Here's how the part is built. I have some questions about the finished solid (model axes, mm). Face numbers are marked on the shaded views. A direction names the side the tool comes from. Round coordinates to 2 decimals unless told otherwise and drop trailing zeros. Order: outer loops, then holes, each group sorted by start corner. A loop starts at its lowest first (then second) coordinate and runs counter-clockwise, first axis right, second up. Notation, with made-up numbers: M 33.25,-40 L 83.25,-40 A28 ccw 83.25,-7 Z; hole C -36.5,15.5 d2. An arc over 180 degrees is marked long. Write each question's results on one line, items separated by ' | '. Start each with the question number.
```python
from build123d import *

# Parameters (mm, degrees)
SKETCH1_R           = 9
SKETCH1_R_2         = 4
BOSS_EXTRUDE1_DEPTH = 5
SKETCH2_W           = 5
SKETCH2_H           = 10
CUT_EXTRUDE3_DEPTH  = 4
CIRPATTERN1_COUNT   = 6


with BuildPart() as part:
    # Sketch1 → Boss-Extrude1 (new body, symmetric)
    with BuildSketch(Plane.XY):
        Circle(SKETCH1_R)
        Circle(SKETCH1_R_2, mode=Mode.SUBTRACT)
    extrude(amount=BOSS_EXTRUDE1_DEPTH, both=True)

    # Sketch2 → Cut-Extrude3 (cut)
    with BuildSketch(Plane(origin=(-9, -17.193061184, 0), x_dir=(0, -1, 0), z_dir=(1, 0, 0))):
        with Locations((-17.193061184, 0)):
            Rectangle(SKETCH2_W, SKETCH2_H)
    cut_extrude3 = extrude(amount=CUT_EXTRUDE3_DEPTH, mode=Mode.SUBTRACT)

    # CirPattern1: Cut-Extrude3 ×6 about axis
    cirpattern1_axis = Axis((0, 0, 0), (0, 0, 1))
    for i in range(1, CIRPATTERN1_COUNT):
        add(cut_extrude3.rotate(cirpattern1_axis, i * 360 / CIRPATTERN1_COUNT), mode=Mode.SUBTRACT)


solid = part.part
```
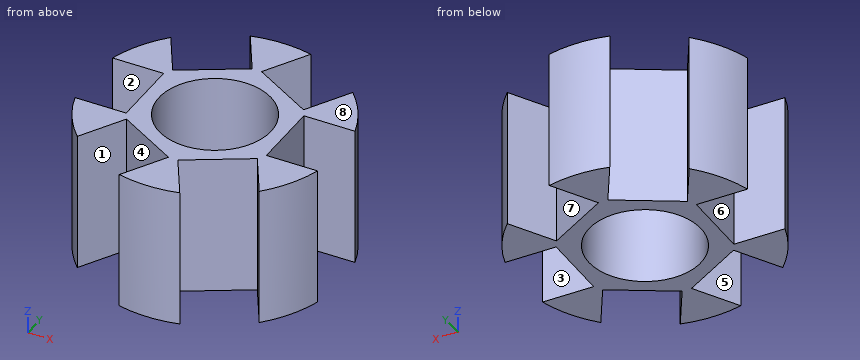
(1) Please list where these lines run through material, in increasing order: line 1 (Y direction, x = 0, z = 1); line 2 (Y direction, x = -0.75, z = 1.75); line 3 (X direction, y = 5, z = -3.5).
(2) On a 3-axis mill with a long thin cutter (end or side, diameter ignored), from which of +Z, -Z, +X, -X, +Y, -Y can I reach the whole of each face in a straight line? I mean the marked faces 1, 2, 3 and 4. Say none if no direction works.
(3) I want a section at B-B on x = 0. Write out the boundary of the cut face in (y, z), and give its area (3 significant figures).
(4) I want a section at A-A on z = 2.5. Write out the boundary of the cut face in (x, y), and give its area (3 significant figures).
(5) I'm going to push flat-ended pins straight in: pin 1 Ø5 at (x, z) = (-1.5, 2) entering from -Y; pin 2 Ø5 at (y, z) = (-3.5, 1.5) entering from +X; pin 3 Ø1.1 at (x, z) = (-6, 1.5) entering from -Y; pin 4 Ø1 at (y, z) = (0.5, -3.5) entering from +X. Where does each tip first touch, or does it pass through?
(6) If we mould it in two halves opening along X, with no side actions, what happens to the marked faces 5, 6, 7 and 8? For each: pulls with the +X half, pulls with the -X half, needs draft (parallel to the pull), parting line crosses it, or undercut.
(7) I want a section at D-D on y = 6. Write out the boundary of the cut face in (x, z).
(8) I want a section at C-C on y = 0. Write out the boundary of the cut face in (x, z), and give its area (3 significant figures).
Solutions:
1) line 1: -9 to -4, 4 to 9 | line 2: -8.97 to -6.3, -5.34 to -3.93, 3.93 to 5.34, 6.3 to 8.97 | line 3: -7.48 to -5.77, -1.34 to 1.34, 5.77 to 7.48
2) face 1: +Z, -Z, -Y | face 2: +Z, -Z, -X | face 3: +Z, -Z, +X | face 4: +Z, -Z
3) outline: M -9,-5 L -4,-5 L -4,5 L -9,5 Z; M 4,-5 L 9,-5 L 9,5 L 4,5 Z | area: 100 mm^2
4) outline: M -8.65,-2.5 A9 ccw -6.49,-6.24 L -4.67,-3.08 L -0.33,-5.58 L -2.16,-8.74 A9 ccw 2.16,-8.74 L 0.33,-5.58 L 4.67,-3.08 L 6.49,-6.24 A9 ccw 8.65,-2.5 L 5,-2.5 L 5,2.5 L 8.65,2.5 A9 ccw 6.49,6.24 L 4.67,3.08 L 0.33,5.58 L 2.16,8.74 A9 ccw -2.16,8.74 L -0.33,5.58 L -4.67,3.08 L -6.49,6.24 A9 ccw -8.65,2.5 L -5,2.5 L -5,-2.5 Z; hole C 0,0 d8 | area: 87.7 mm^2
5) pin 1: y = -9 | pin 2: x = 8.65 | pin 3: y = -6.24 | pin 4: x = 5
6) face 5: undercut | face 6: pulls with the -X half | face 7: undercut | face 8: needs draft
7) outline: M -6.71,-5 L -6.35,-5 L -6.35,5 L -6.71,5 Z; M -0.58,-5 L 0.58,-5 L 0.58,5 L -0.58,5 Z; M 6.35,-5 L 6.71,-5 L 6.71,5 L 6.35,5 Z
8) outline: M -5,-5 L -4,-5 L -4,5 L -5,5 Z; M 4,-5 L 5,-5 L 5,5 L 4,5 Z | area: 20.0 mm^2
